The drawing under review shows one solid part. Ordinate dimensions are in mm from its lowest x, y, z. Round coordinates to 2 decimals unless told otherwise and drop trailing zeros. Loops run counter-clockwise (first coordinate to the right, second up) from the corner with the lowest first, then second, coordinate; pieces in that order, holes last. Notation, with made-up numbers: (64, -21.75) - (73, -21.75) arc R27 cw to (73, -0.75) - close; hole circle Ø2 at (68, -19). An arc over 180 degrees is marked (long way). Answer as CSV lines item,"result".
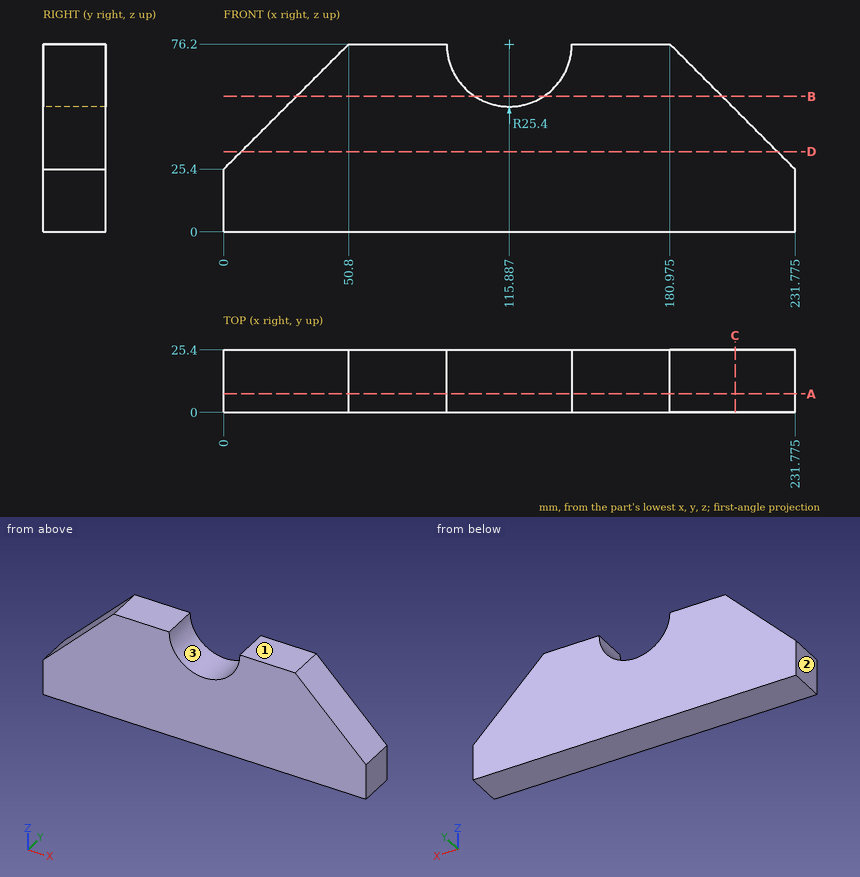
1. Take a section at D-D (z = 32.5). State the section outline as (x, y) points (1 decimal), plus the area to 3 significant figures.
Numbers:
outline,"(7.1, 0) - (224.7, 0) - (224.7, 25.4) - (7.1, 25.4) - close"
area,"5,530 mm²"
2. Take a section at C-C (x = 207.5). State the section outline as (y, z) points (1 decimal).
Numbers:
outline,"(0, 0) - (25.4, 0) - (25.4, 49.7) - (0, 49.7) - close"
3. Take a section at B-B (z = 55). State the section outline as (x, y) points (1 decimal).
Numbers:
outline,"(29.6, 0) - (101.9, 0) - (101.9, 25.4) - (29.6, 25.4) - close; (129.9, 0) - (202.2, 0) - (202.2, 25.4) - (129.9, 25.4) - close"
4. Clearance check with a flat-ended pin moving along its axis: pin 1 (1 mm diameter, centred on y = 15, z = 68, fed in from +X) (1 decimal). State where the tip first meets the part, or that it passes through.
Numbers:
pin 1,"stops at x = 189.7"
5. Take a section at A-A (y = 7.5). State the section outline as (x, z) points (1 decimal), plus the area to 3 significant figures.
Numbers:
outline,"(0, 0) - (231.8, 0) - (231.8, 25.4) - (181, 76.2) - (141.3, 76.2) arc R25.4 cw to (90.5, 76.2) - (50.8, 76.2) - (0, 25.4) - close"
area,"14,100 mm²"
6. Draft analysis for pull direction X (two halves, no side actions). For the marked faces 1, 2 and 3, state which applies: +X half, -X half, draft (parallel to the pull), parting line (faces both ways), or undercut.
Numbers:
face 1,"draft"
face 2,"-X half"
face 3,"undercut"
7. Wall thickness on probe 1 along X at (y, z) = (10.5, 60.5) (1 decimal); probe 2 along Z at (x, y) = (116.5, 24.25); probe 3 along X at (y, z) = (14.75, 46) (1 decimal): over which ranges is each line inside the solid? List them lowest first.
Numbers:
probe 1,"x = 35.1 to 95.9, 135.9 to 196.7"
probe 2,"z = 0 to 50.81"
probe 3,"x = 20.6 to 211.2"
